Work out the finished part from the listing and answer in its coordinate system (mm). Coordinates: 2 decimals unless noted, no trailing zeros. Loops run counter-clockwise (first coordinate to the right, second up) from the corner with the lowest first, then second, coordinate; pieces in that order, holes last. Notation, with made-up numbers: (53.5, -0.5) -> (103.5, -0.5) arc R10 ccw to (103.5, 3.5) -> close; hole circle Ø7 at (18, -12.75). An arc over 180 degrees is marked (long way). Use a Markdown table: item, result.
from build123d import *

# Parameters (mm, degrees)
SKETCH_1_R      = 1.35
SKETCH_1_R_2    = 1.3
SKETCH_1_W      = 12.200420097
SKETCH_1_H      = 23.000703054
EXTRUDE_1_DEPTH = 3


with BuildPart() as part:
    # 草图1 → 凸台-拉伸1 (new body)
    with BuildSketch(Plane.XZ.offset(0.906223555)):
        with BuildLine():
            Line((-25.648543234, 0), (18.351102305, 0))
            ThreePointArc((18.351102305, 0), (20.472422649, 0.878679656), (21.351102305, 3))
            Line((21.351102305, 3), (21.351102305, 46.999948986))
            ThreePointArc((21.351102305, 46.999948986), (20.472422649, 49.12126933), (18.351102305, 49.999948986))
            Line((18.351102305, 49.999948986), (-25.648543234, 49.999948986))
            ThreePointArc((-25.648543234, 49.999948986), (-27.769863578, 49.12126933), (-28.648543234, 46.999948986))
            Line((-28.648543234, 46.999948986), (-28.648543234, 3))
            ThreePointArc((-28.648543234, 3), (-27.769863578, 0.878679656), (-25.648543234, 0))
        make_face()
        with Locations(Location((18.351102305, 46.999948986, 0), (0, 0, 90))):
            Circle(SKETCH_1_R, mode=Mode.SUBTRACT)
        with Locations(Location((-25.648543234, 3, 0), (0, 0, 90))):
            Circle(SKETCH_1_R, mode=Mode.SUBTRACT)
        with Locations(Location((-25.648543234, 46.999948986, 0), (0, 0, 90))):
            Circle(SKETCH_1_R, mode=Mode.SUBTRACT)
        with Locations(Location((18.351102305, 3, 0), (0, 0, 90))):
            Circle(SKETCH_1_R, mode=Mode.SUBTRACT)
        with Locations(Location((5.870533839, 25.026548182, 0), (0, 0, 90))):
            Circle(SKETCH_1_R_2, mode=Mode.SUBTRACT)
        with Locations(Location((-13.129904617, 24.994501462, 0), (0, 0, 90))):
            Circle(SKETCH_1_R_2, mode=Mode.SUBTRACT)
        with Locations((-3.648510984, 25.000507943)):
            Rectangle(SKETCH_1_W, SKETCH_1_H, mode=Mode.SUBTRACT)
    extrude(amount=-EXTRUDE_1_DEPTH)


solid = part.part
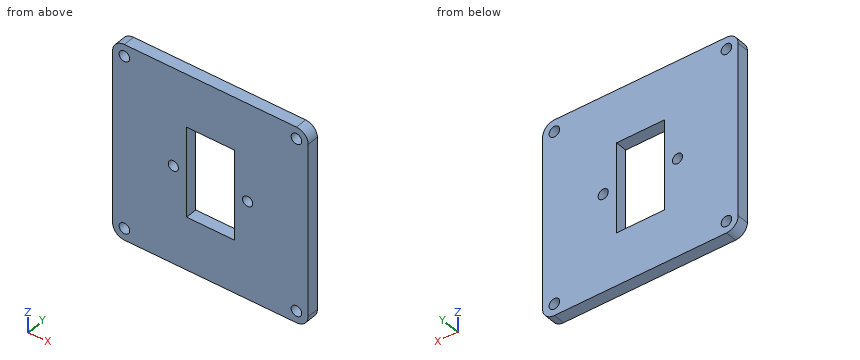
Q1. Consider line 1 (X direction, y = 1.8, z = 25); line 2 (X direction, y = 0.25, z = 3); line 3 (X direction, y = 0.4, z = 31). Determine where each line is inside the solid, lowest interval first. Write a range as [from, to].
Solved:
| item | result |
|---|---|
| line 1 | [-28.65, -14.43], [-11.83, -9.75], [2.45, 4.57], [7.17, 21.35] |
| line 2 | [-28.65, -27], [-24.3, 17], [19.7, 21.35] |
| line 3 | [-28.65, -9.75], [2.45, 21.35] |
Q2. Section C-C on y = -0.05 is taken. Determine the outline of the cut face in (x, z), and give its area (3 significant figures).
Solved:
| item | result |
|---|---|
| outline | (-28.65, 3) arc R3 ccw to (-25.65, 0) -> (18.35, 0) arc R3 ccw to (21.35, 3) -> (21.35, 47) arc R3 ccw to (18.35, 50) -> (-25.65, 50) arc R3 ccw to (-28.65, 47) -> close; hole circle Ø2.7 at (-25.65, 3); hole circle Ø2.7 at (-25.65, 47); hole circle Ø2.6 at (-13.13, 24.99); hole (-9.75, 13.5) -> (2.45, 13.5) -> (2.45, 36.5) -> (-9.75, 36.5) -> close; hole circle Ø2.6 at (5.87, 25.03); hole circle Ø2.7 at (18.35, 3); hole circle Ø2.7 at (18.35, 47) |
| area | 2,180 mm² |
Q3. Given pin 1 Ø2 at (x, z) = (5.87, 25.03) entering from +Y; pin 2 Ø3.5 at (x, z) = (-25.65, 3) entering from -Y, each flat-ended and moving along its own axis, determine where each tip first touches the part or whether it passes through.
Solved:
| item | result |
|---|---|
| pin 1 | through |
| pin 2 | y = -0.91 |
Q4. Section B-B on z = 18 is taken. Determine the outline of the cut face in (x, y), and give its area (3 significant figures).
Solved:
| item | result |
|---|---|
| outline | (-28.65, -0.91) -> (-9.75, -0.91) -> (-9.75, 2.09) -> (-28.65, 2.09) -> close; (2.45, -0.91) -> (21.35, -0.91) -> (21.35, 2.09) -> (2.45, 2.09) -> close |
| area | 113 mm² |
Q5. Section A-A on x = -3 is taken. Determine the outline of the cut face in (y, z), and give its area (3 significant figures).
Solved:
| item | result |
|---|---|
| outline | (-0.91, 0) -> (2.09, 0) -> (2.09, 13.5) -> (-0.91, 13.5) -> close; (-0.91, 36.5) -> (2.09, 36.5) -> (2.09, 50) -> (-0.91, 50) -> close |
| area | 81.0 mm² |
